Geometry check sheet. Reference: the model listing, model coordinates, mm. A direction names the side the tool comes from. Coordinates: 2 decimals unless noted, no trailing zeros. Write each loop counter-clockwise with the first axis right and the second up, starting at its lowest first coordinate (ties: lowest second). Pieces come first, ordered by that corner, then holes. Notation, with made-up numbers: (-20.75, -33.5) - (-15.75, -33.5) arc R21 ccw to (-15.75, -15.5) - close; hole circle Ø3 at (63, 30). An arc over 180 degrees is marked (long way). Answer as a JSON object with one key per item and string values. Group by question number.
from build123d import *

# Parameters (mm, degrees)
F0_R     = 4
F1_DEPTH = 2
F2_R     = 1
F3_R     = 2.15
F4_DEPTH = 2
F5_R     = 4
F6_DEPTH = 2
F7_R     = 1
F8_R     = 2
F9_DEPTH = 6


with BuildPart() as f1:
    # F0 (on Front) → F1 (new body)
    with BuildSketch(Plane.XZ):
        Circle(F0_R)
    extrude(amount=F1_DEPTH)

    # F2
    f2_edges = [f1.edges().sort_by_distance(p)[0] for p in [
        (-4, -2, 0),
    ]]
    fillet(f2_edges, radius=F2_R)

    # F3 (on face) → F4 (join)
    with BuildSketch(Plane(origin=(0, 0, 0), x_dir=(-1, 0, 0), z_dir=(0, 1, 0))):
        Circle(F3_R)
    extrude(amount=F4_DEPTH)

    # F5 (on face) → F6 (join)
    with BuildSketch(Plane(origin=(0, 2, 0), x_dir=(-1, 0, 0), z_dir=(0, 1, 0))):
        Circle(F5_R)
    extrude(amount=F6_DEPTH)

    # F7
    f7_edges = [f1.edges().sort_by_distance(p)[0] for p in [
        (4, 4, 0),
    ]]
    fillet(f7_edges, radius=F7_R)

    # F8 (on face) → F9 (cut)
    with BuildSketch(Plane(origin=(0, 4, 0), x_dir=(-1, 0, 0), z_dir=(0, 1, 0))):
        Circle(F8_R)
    extrude(amount=-F9_DEPTH, mode=Mode.SUBTRACT)


solid = f1.part
(1) Gauge pin test, flat ends, axial feed: pin 1 (1 mm diameter, centred on y = -0.5, z = -3, fed in from +X); pin 2 (3 mm diameter, centred on x = 0, z = 0, fed in from -Y). Record the tip position at first contact, or that the pin passes through.
(2) Set-up check for faces 1 (the face through (0.867, 2.493, -3.905)), 2 (the face through (2, 0, -2)): record each of +Z, -Z, +X, -X, +Y, -Y from which the full face is reachable in a straight line by a thin tool's end or side.
(3) Section check C-C (y = 2.35). Record the cut outline in (x, z).
(4) Section check B-B (z = 0). Record the cut outline in (x, y).
(5) Material ranges on L1, parallel to Y at x = -2.75, z = -1; L2, parallel to Y at x = 3.75, z = -0.5; L3, parallel to X at y = 3.2, z = 0.5, recorded low to high. Write a range as [from, to].
(6) Section check A-A (x = 0). Record the cut outline in (y, z).
(7) Section check D-D (y = 1.35). Record the cut outline in (x, z).
(8) Draft check along Y on faces 3 (the face through (1, -2, -2)), 4 (the face through (2.15, 0.99, 0.09)), 5 (the face through (-1, 4, -2)), 6 (the face through (0.434, 1.042, -1.952)). Enter one of: +Y half, -Y half, draft (parallel to the pull), parting line (faces both ways), or undercut.
Conclusion:
{
 "1": {"pin 1": "stops at x = 3.12", "pin 2": "passes through"},
 "2": {"face 1": "+Y, -Y", "face 2": "none"},
 "3": {"outline": "circle Ø8 at (0, 0); hole circle Ø4 at (0, 0)"},
 "4": {"outline": "(-4, -1) arc R1 ccw to (-3, -2) - (-2, -2) - (-2, 4) - (-3, 4) arc R1 ccw to (-4, 3) - (-4, 2) - (-2.15, 2) - (-2.15, 0) - (-4, 0) - close; (2, -2) - (3, -2) arc R1 ccw to (4, -1) - (4, 0) - (2.15, 0) - (2.15, 2) - (4, 2) - (4, 3) arc R1 ccw to (3, 4) - (2, 4) - close"},
 "5": {"L1": "y = [-2, 0], [2, 4]", "L2": "y = [-1.62, 0], [2, 3.62]", "L3": "x = [-3.95, -1.94], [1.94, 3.95]"},
 "6": {"outline": "(-2, -3) arc R1 ccw to (-1, -4) - (0, -4) - (0, -2.15) - (2, -2.15) - (2, -4) - (3, -4) arc R1 ccw to (4, -3) - (4, -2) - (-2, -2) - close; (-2, 2) - (4, 2) - (4, 3) arc R1 ccw to (3, 4) - (2, 4) - (2, 2.15) - (0, 2.15) - (0, 4) - (-1, 4) arc R1 ccw to (-2, 3) - close"},
 "7": {"outline": "circle Ø4.3 at (0, 0); hole circle Ø4 at (0, 0)"},
 "8": {"face 3": "-Y half", "face 4": "undercut", "face 5": "+Y half", "face 6": "draft"}
}
